```python
from build123d import *

# Parameters (mm, degrees)
SKETCH1_W           = 70
SKETCH1_H           = 70
SKETCH1_W_2         = 64
SKETCH1_H_2         = 64
BOSS_EXTRUDE1_DEPTH = 1000
FILLET1_R           = 5
SKETCH2_R           = 3
CUT_EXTRUDE1_DEPTH  = 70
SKETCH4_R           = 3
CUT_EXTRUDE2_DEPTH  = 70


with BuildPart() as part:
    # Sketch1 → Boss-Extrude1 (new body)
    with BuildSketch(Plane.XY):
        with Locations((35, 35)):
            Rectangle(SKETCH1_W, SKETCH1_H)
        with Locations((35, 35)):
            Rectangle(SKETCH1_W_2, SKETCH1_H_2, mode=Mode.SUBTRACT)
    extrude(amount=BOSS_EXTRUDE1_DEPTH)

    # Fillet1
    fillet1_edges = [part.edges().sort_by_distance(p)[0] for p in [
        (3, 67, 500),
        (3, 3, 500),
        (67, 3, 500),
        (67, 67, 500),
        (0, 70, 500),
        (70, 70, 500),
        (70, 0, 500),
        (0, 0, 500),
    ]]
    fillet(fillet1_edges, radius=FILLET1_R)

    # Sketch2 → Cut-Extrude1 (cut)
    with BuildSketch(Plane(origin=(0, 70, 0), x_dir=(1, 0, 0), z_dir=(0, 1, 0))):
        with Locations(Location((35, -965, 0), (0, 0, 270))):
            Circle(SKETCH2_R)
        with Locations(Location((35, -35, 0), (0, 0, 270))):
            Circle(SKETCH2_R)
    extrude(amount=-CUT_EXTRUDE1_DEPTH, mode=Mode.SUBTRACT)

    # Sketch4 → Cut-Extrude2 (cut)
    with BuildSketch(Plane.XZ):
        with Locations(Location((54.09, 515.91, 0), (0, 0, 270))):
            Circle(SKETCH4_R)
        with Locations(Location((54.09, 484.09, 0), (0, 0, 270))):
            Circle(SKETCH4_R)
    extrude(amount=-CUT_EXTRUDE2_DEPTH, mode=Mode.SUBTRACT)


solid = part.part
```
Source: CAD feature listing. Evaluate the final solid. Frame: model axes, mm. A direction names the side the tool comes from. Coordinates: 2 decimals unless noted, no trailing zeros. Loops run counter-clockwise (first coordinate to the right, second up) from the corner with the lowest first, then second, coordinate; pieces in that order, holes last. Notation, with made-up numbers: M 14.5,-20.75 L 52.5,-20.75 A24 ccw 52.5,-1.75 Z; hole C 36,-17 d6. An arc over 180 degrees is marked long. Put each result on its own line as item: value. Start each with the question number.
1) Cut plane A-A on y = 24. Return the cut outline in (x, z).
2) Ray query, L1, parallel to Z at x = 54, y = 68; L2, parallel to Y at x = 45, z = 678. Return the intervals inside material, ascending. Write a range as from..to.
3) Cut plane B-B on z = 585. Return the cut outline in (x, y).
4) Pull-direction query (X, two-part tool) for faces 3 (the face through (0, 35, 493)), 4 (the face through (70, 35, 493)), 5 (the face through (35, 67, 493)), 6 (the face through (35, 70, 493)); classes: pulls with the +X half, pulls with the -X half, needs draft (parallel to the pull), parting line crosses it, or undercut.
5) Reachability of faces 1 (the face through (3, 35, 493)), 2 (the face through (32, 1, 0)) from +Z, -Z, +X, -X, +Y, -Y: full face, straight path, thin tool, end or side. Return the list, or none.
6) Contact query for flat-ended pins moving along their axis: pin 1 Ø9.5 at (x, z) = (54.09, 515.91) entering from -Y; pin 2 Ø5.5 at (x, z) = (54.09, 484.09) entering from -Y. Output: stop coordinate, or through.
The answers:
1. outline: M 0,0 L 3,0 L 3,1000 L 0,1000 Z; M 67,0 L 70,0 L 70,1000 L 67,1000 Z
2. L1: z = 0..481.09, 487.09..512.91, 518.91..1000
2. L2: y = 0..3, 67..70
3. outline: M 0,5 A5 ccw 5,0 L 65,0 A5 ccw 70,5 L 70,65 A5 ccw 65,70 L 5,70 A5 ccw 0,65 Z; hole M 3,8 A5 ccw 8,3 L 62,3 A5 ccw 67,8 L 67,62 A5 ccw 62,67 L 8,67 A5 ccw 3,62 Z
4. face 3: pulls with the -X half
4. face 4: pulls with the +X half
4. face 5: undercut
4. face 6: needs draft
5. face 1: +Z, -Z
5. face 2: -Z, +X, -X, +Y, -Y
6. pin 1: stops at y = 0
6. pin 2: passes through
